Read the model definition and answer for the solid it produces. Units are mm, in the model's axes. A direction names the side the tool comes from. Coordinates: 2 decimals unless noted, no trailing zeros. Order: outer loops, then holes, each group sorted by start corner. A loop starts at its lowest first (then second) coordinate and runs counter-clockwise, first axis right, second up. Notation, with made-up numbers: (30, 70) - (57, 70) arc R13 cw to (57, 89) - close; hole circle Ø1 at (-38, 59.5). An arc over 180 degrees is marked (long way). Use one line per item in the form item = value.
```python
from build123d import *

# Parameters (mm, degrees)
F0_W      = 38.1
F0_H      = 31.75
F1_DEPTH  = 12.7
F2_R      = 3.175
F3_DEPTH  = 31.751
F4_W      = 6.48
F4_H      = 6.48
F5_DEPTH  = 3.302
F6_W      = 76.2
F6_H      = 12.7
F7_DEPTH  = 19.05
F9_DEPTH  = 6.35
F10_W     = 12.7
F10_H     = 12.7
F11_DEPTH = 6.35
F12_R     = 5.08
F13_R     = 3
F14_DEPTH = 31.751
F15_R     = 3
F16_DEPTH = 5.5
F17_R     = 5.08


with BuildPart() as f1:
    # F0 (on Top) → F1 (new body, symmetric)
    with BuildSketch(Plane.XY):
        Rectangle(F0_W, F0_H)
        Polygon((12.954, 9.779), (12.954, -9.779), (-12.954, -9.779), (-12.954, 9.779), (-5.842, 9.779), (-5.842, 3.937), (6.35, 3.937), (6.35, 9.779), align=None, mode=Mode.SUBTRACT)
    extrude(amount=F1_DEPTH, both=True)

    # F2 (on face) → F3 (cut, through all)
    with BuildSketch(Plane.XZ.offset(15.875)):
        Circle(F2_R)
    extrude(amount=-F3_DEPTH, mode=Mode.SUBTRACT)

    # F4 (on face) → F5 (cut)
    with BuildSketch(Plane.XZ.offset(15.875)):
        Rectangle(F4_W, F4_H)
    extrude(amount=-F5_DEPTH, mode=Mode.SUBTRACT)

    # F6 (on face) → F7 (join)
    with BuildSketch(Plane.XY.offset(12.7)):
        with Locations((57.15, -9.525)):
            Rectangle(F6_W, F6_H)
    extrude(amount=-F7_DEPTH)

    # F8 (on face) → F9 (join)
    with BuildSketch(Plane.XZ.offset(15.875)):
        Polygon((19.05, -6.35), (19.05, -12.7), (44.45, -6.35), align=None)
    extrude(amount=-F9_DEPTH)

    # F10 (on face) → F11 (join)
    with BuildSketch(Plane.XY.offset(12.7)):
        with Locations((25.654, -9.525)):
            Rectangle(F10_W, F10_H)
        with Locations((78.994, -9.525)):
            Rectangle(F10_W, F10_H)
    extrude(amount=F11_DEPTH)

    # F12
    f12_edges = [f1.edges().sort_by_distance(p)[0] for p in [
        (19.304, -9.525, 19.05),
        (32.004, -9.525, 19.05),
        (72.644, -9.525, 19.05),
        (85.344, -9.525, 19.05),
    ]]
    fillet(f12_edges, radius=F12_R)

    # F13 (on face) → F14 (cut, through all)
    with BuildSketch(Plane.XZ.offset(15.875)):
        with Locations((25.653916178, 11.4300000005)):
            Circle(F13_R)
        with Locations((79.0242652024, 11.4300601041)):
            Circle(F13_R)
    extrude(amount=-F14_DEPTH, mode=Mode.SUBTRACT)

    # F15 (on face) → F16 (cut)
    with BuildSketch(Plane(origin=(0, -3.175, 0), x_dir=(-1, 0, 0), z_dir=(0, 1, 0))):
        Polygon((-84.0242652024, 8.5433087581), (-79.0242652024, 5.6565574122), (-74.0242652024, 8.5433087581), (-74.0242652024, 14.31681145), (-79.0242652024, 17.203562796), (-84.0242652024, 14.31681145), align=None)
        with Locations((-79.0242652024, 11.4300601041)):
            Circle(F15_R, mode=Mode.SUBTRACT)
        Polygon((-30.653916178, 8.5432486545), (-25.653916178, 5.6564973086), (-20.653916178, 8.5432486545), (-20.653916178, 14.3167513464), (-25.653916178, 17.2035026924), (-30.653916178, 14.3167513464), align=None)
        with Locations((-25.653916178, 11.4300000005)):
            Circle(F15_R, mode=Mode.SUBTRACT)
    extrude(amount=-F16_DEPTH, mode=Mode.SUBTRACT)

    # F17
    f17_edges = [f1.edges().sort_by_distance(p)[0] for p in [
        (95.25, -9.525, 12.7),
        (95.25, -9.525, -6.35),
    ]]
    fillet(f17_edges, radius=F17_R)


solid = f1.part
```
(1) Which of the six approach directions +Z, -Z, +X, -X, +Y, -Y give full straight-line access (tool end or side, diameter ignored) to faces 1 (the cylindrical face through (74.09, -9.44, 17.52)), 2 (the flat face through (28.12, -5.89, 15.78)), 3 (the flat face through (-2, -12.573, -3)), 4 (the flat face through (-12.954, 0, 0))?
Answer list:
face_1 = +Z, +Y, -Y
face_2 = +Y
face_3 = -Y
face_4 = +Z, -Z
(2) Section D-D, the plane y = 13 is taken. Write down the section's boundary in (x, z) (3 decimals).
Answer list:
outline = (-19.05, -12.7) - (19.05, -12.7) - (19.05, 12.7) - (-19.05, 12.7) - close; hole circle Ø6.35 at (0, 0)
(3) Straight lines are drawn through the part: L1, parallel to X at y = 5, z = 3.5; L2, parallel to X at y = -3.5, z = 4; L3, parallel to Y at x = -5.5, z = -5.5 (3 decimals). For each, find the intervals that lie inside material, in ascending order.
Answer list:
L1 = -19.05 to -12.95, -5.84 to 6.35, 12.95 to 19.05
L2 = -19.05 to -12.95, 12.95 to 95.25
L3 = -15.875 to -9.779, 3.937 to 15.875
(4) Section A-A, the plane z = 0 is taken. Write down the section's boundary in (x, y) (3 decimals), then the cut area to 3 significant figures.
Answer list:
outline = (-19.05, -15.875) - (-3.24, -15.875) - (-3.24, -12.573) - (-3.175, -12.573) - (-3.175, -9.779) - (-12.954, -9.779) - (-12.954, 9.779) - (-5.842, 9.779) - (-5.842, 3.937) - (-3.175, 3.937) - (-3.175, 15.875) - (-19.05, 15.875) - close; (3.175, -12.573) - (3.24, -12.573) - (3.24, -15.875) - (95.25, -15.875) - (95.25, -3.175) - (19.05, -3.175) - (19.05, 15.875) - (3.175, 15.875) - (3.175, 3.937) - (6.35, 3.937) - (6.35, 9.779) - (12.954, 9.779) - (12.954, -9.779) - (3.175, -9.779) - close
area = 1,630 mm2
(5) Section C-C, the plane x = 0 is taken. Write down the section's boundary in (y, z) (3 decimals).
Answer list:
outline = (-15.875, -12.7) - (-9.779, -12.7) - (-9.779, -3.175) - (-12.573, -3.175) - (-12.573, -3.24) - (-15.875, -3.24) - close; (-15.875, 3.24) - (-12.573, 3.24) - (-12.573, 3.175) - (-9.779, 3.175) - (-9.779, 12.7) - (-15.875, 12.7) - close; (3.937, -12.7) - (15.875, -12.7) - (15.875, -3.175) - (3.937, -3.175) - close; (3.937, 3.175) - (15.875, 3.175) - (15.875, 12.7) - (3.937, 12.7) - close
(6) The mould has two halves that part along X. Classify faces 5 (the flat face through (31.57, -12.74, -9.57)), 6 (the flat face through (37, -15.875, 3)), 7 (the cylindrical face through (20.75, -9.44, 17.52)), 8 (the flat face through (3, -9.779, -3)): +X half, -X half, draft (parallel to the pull), parting line (faces both ways), or undercut.
Answer list:
face_5 = +X half
face_6 = draft
face_7 = -X half
face_8 = undercut
(7) Given pin 1 Ø3.5 at (x, z) = (79.02, 11.43) entering from -Y; pin 2 Ø12 at (x, z) = (27, -0.5) entering from +Y (3 decimals); pin 3 Ø8 at (x, y) = (6.5, 6) entering from +Z; pin 4 Ø12 at (x, y) = (78.5, -1.5) entering from -Z, each flat-ended and moving along its own axis, determine where each tip first touches the part or whether it passes through.
Answer list:
pin_1 = through
pin_2 = -3.175
pin_3 = 12.7
pin_4 = -6.35
(8) Section B-B, the plane y = 6 is taken. Write down the section's boundary in (x, z) (3 decimals), then the cut area to 3 significant figures.
Answer list:
outline = (-19.05, -12.7) - (-12.954, -12.7) - (-12.954, 12.7) - (-19.05, 12.7) - close; (-5.842, -12.7) - (6.35, -12.7) - (6.35, 12.7) - (-5.842, 12.7) - close; (12.954, -12.7) - (19.05, -12.7) - (19.05, 12.7) - (12.954, 12.7) - close; hole circle Ø6.35 at (0, 0)
area = 588 mm2
